```python
from build123d import *

# Parameters (mm, degrees)
SKETCH1_R           = 10.8
BOSS_EXTRUDE1_DEPTH = 13
SKETCH2_R           = 14.5
BOSS_EXTRUDE2_DEPTH = 9
SKETCH3_R           = 16.3
BOSS_EXTRUDE3_DEPTH = 6.9
SKETCH4_R           = 19.5
BOSS_EXTRUDE4_DEPTH = 7
FILLET1_R           = 2
SKETCH5_W           = 29.75
SKETCH5_H           = 32.65
BOSS_EXTRUDE5_DEPTH = 41.5


with BuildPart() as part:
    # Sketch1 → Boss-Extrude1 (new body)
    with BuildSketch(Plane.XY):
        Circle(SKETCH1_R)
    extrude(amount=BOSS_EXTRUDE1_DEPTH)

    # Sketch2 → Boss-Extrude2 (add)
    with BuildSketch(Plane(origin=(0, 0, 0), x_dir=(-1, 0, 0), z_dir=(0, 0, -1))):
        Circle(SKETCH2_R)
    extrude(amount=BOSS_EXTRUDE2_DEPTH)

    # Sketch3 → Boss-Extrude3 (add)
    with BuildSketch(Plane(origin=(0, 0, -9), x_dir=(-1, 0, 0), z_dir=(0, 0, -1))):
        Circle(SKETCH3_R)
    extrude(amount=BOSS_EXTRUDE3_DEPTH)

    # Sketch4 → Boss-Extrude4 (add)
    with BuildSketch(Plane(origin=(0, 0, -15.9), x_dir=(-1, 0, 0), z_dir=(0, 0, -1))):
        Circle(SKETCH4_R)
    extrude(amount=BOSS_EXTRUDE4_DEPTH)

    # Fillet1
    fillet1_edges = [part.edges().sort_by_distance(p)[0] for p in [
        (19.5, 0, -15.9),
        (19.5, 0, -22.9),
    ]]
    fillet(fillet1_edges, radius=FILLET1_R)

    # Sketch5 → Boss-Extrude5 (add)
    with BuildSketch(Plane.XY.offset(13)):
        Rectangle(SKETCH5_W, SKETCH5_H)
    extrude(amount=BOSS_EXTRUDE5_DEPTH)


solid = part.part
```
Part model, mm, in its own coordinate system. A direction names the side the tool comes from. Give positions to 0.01 mm unless a question says otherwise; leave off trailing zeros. Write each loop counter-clockwise with the first axis right and the second up, starting at its lowest first coordinate (ties: lowest second). Pieces come first, ordered by that corner, then holes. Notation, with made-up numbers: (66, 13.5) -> (97, 13.5) arc R23 ccw to (97, 42.5) -> close; hole circle Ø1 at (-14.75, 31.5). An arc over 180 degrees is marked (long way). Put each result on its own line as item: value. Start each with the question number.
Item 1: Cut at A-A (y = 0). List the corners of the cut face in (x, z) (3 decimals).
Item 2: Which spindle directions (+Z, -Z, +X, -X, +Y, -Y) get a long thin tool onto all of the face, cutting with end or side? Do faces 1 (the face through (-14.875, 0, 33)), 2 (the face through (14.875, 0, 33)), 3 (the face through (0, 16.325, 33)), 4 (the face through (0, 11, 0)). Say none if no direction does.
Item 3: Pull direction Z, two halves, no side cores. Call faces 5 (the face through (0, 0, -22.9)), 6 (the face through (0, -16.325, 33)), 7 (the face through (0, 11, 13)), 8 (the face through (-2.341, -10.543, 6.409)): pulls with the +Z half, pulls with the -Z half, needs draft (parallel to the pull), parting line crosses it, or undercut.
Item 4: Cut at D-D (z = 35.5). List the corners of the cut face in (x, y) (3 decimals).
Item 5: Cut at B-B (x = 0). List the corners of the cut face in (y, z) (3 decimals), then the cut area to 3 significant figures.
Item 6: Wall check: L1, parallel to Z at x = 7, y = -10.5; L2, parallel to Z at x = 0, y = -15; L3, parallel to Y at x = -4, z = 36 (3 decimals). Give the ranges that are in metal, low to high. Write a range as [from, to].
Item 7: Cut at C-C (z = -11.5). List the corners of the cut face in (x, y).
Item 8: Pin check, flat tips, straight feed: pin 1 Ø9 at (x, z) = (-7, 34.5) entering from +Y (3 decimals); pin 2 Ø1.5 at (y, z) = (1.5, 4.5) entering from +X; pin 3 Ø1 at (y, z) = (4.5, 28) entering from +X (3 decimals). Stop position of each tip, or through.
Answer list:
1. outline: (-19.5, -20.9) arc R2 ccw to (-17.5, -22.9) -> (17.5, -22.9) arc R2 ccw to (19.5, -20.9) -> (19.5, -17.9) arc R2 ccw to (17.5, -15.9) -> (16.3, -15.9) -> (16.3, -9) -> (14.5, -9) -> (14.5, 0) -> (10.8, 0) -> (10.8, 13) -> (14.875, 13) -> (14.875, 54.5) -> (-14.875, 54.5) -> (-14.875, 13) -> (-10.8, 13) -> (-10.8, 0) -> (-14.5, 0) -> (-14.5, -9) -> (-16.3, -9) -> (-16.3, -15.9) -> (-17.5, -15.9) arc R2 ccw to (-19.5, -17.9) -> close
2. face 1: +Z, -X, +Y, -Y
2. face 2: +Z, +X, +Y, -Y
2. face 3: +Z, +X, -X, +Y
2. face 4: none
3. face 5: pulls with the -Z half
3. face 6: needs draft
3. face 7: undercut
3. face 8: undercut
4. outline: (-14.875, -16.325) -> (14.875, -16.325) -> (14.875, 16.325) -> (-14.875, 16.325) -> close
5. outline: (-19.5, -20.9) arc R2 ccw to (-17.5, -22.9) -> (17.5, -22.9) arc R2 ccw to (19.5, -20.9) -> (19.5, -17.9) arc R2 ccw to (17.5, -15.9) -> (16.3, -15.9) -> (16.3, -9) -> (14.5, -9) -> (14.5, 0) -> (10.8, 0) -> (10.8, 13) -> (16.325, 13) -> (16.325, 54.5) -> (-16.325, 54.5) -> (-16.325, 13) -> (-10.8, 13) -> (-10.8, 0) -> (-14.5, 0) -> (-14.5, -9) -> (-16.3, -9) -> (-16.3, -15.9) -> (-17.5, -15.9) arc R2 ccw to (-19.5, -17.9) -> close
5. area: 2,390 mm2
6. L1: z = [-22.9, 0], [13, 54.5]
6. L2: z = [-22.9, -9], [13, 54.5]
6. L3: y = [-16.325, 16.325]
7. outline: circle Ø32.6 at (0, 0)
8. pin 1: stops at y = 16.325
8. pin 2: stops at x = 10.77
8. pin 3: stops at x = 14.875
